Input: part model. Units: mm. Frame: model coordinates. Give positions to 0.01 mm unless a question says otherwise; leave off trailing zeros. Loops run counter-clockwise (first coordinate to the right, second up) from the corner with the lowest first, then second, coordinate; pieces in that order, holes last. Notation, with made-up numbers: (7, 4) -> (20, 4) arc R21 cw to (20, 33) -> close; hole circle Ø9 at (73.5, -12.75). An arc over 180 degrees is marked (long way). Use CSV: the item, a comma, the result in double quotes.
```python
from build123d import *

# Parameters (mm, degrees)
SKETCH1_R           = 4.5
BOSS_EXTRUDE1_DEPTH = 4.3
SKETCH2_R           = 3.9
CUT_EXTRUDE1_DEPTH  = 5.3
CHAMFER1_SIZE       = 0.2


with BuildPart() as part:
    # Sketch1 → Boss-Extrude1 (new body)
    with BuildSketch(Plane(origin=(0, 0, 0), x_dir=(1, 0, 0), z_dir=(0, 1, 0))):
        Circle(SKETCH1_R)
    extrude(amount=BOSS_EXTRUDE1_DEPTH)

    # Sketch2 → Cut-Extrude1 (cut, through all)
    with BuildSketch(Plane(origin=(0, 4.3, 0), x_dir=(1, 0, 0), z_dir=(0, 1, 0))):
        Circle(SKETCH2_R)
    extrude(amount=-CUT_EXTRUDE1_DEPTH, mode=Mode.SUBTRACT)

    # Chamfer1
    chamfer1_edges = [part.edges().sort_by_distance(p)[0] for p in [
        (-4.5, 0, 0),
    ]]
    chamfer(chamfer1_edges, length=CHAMFER1_SIZE)


solid = part.part
```
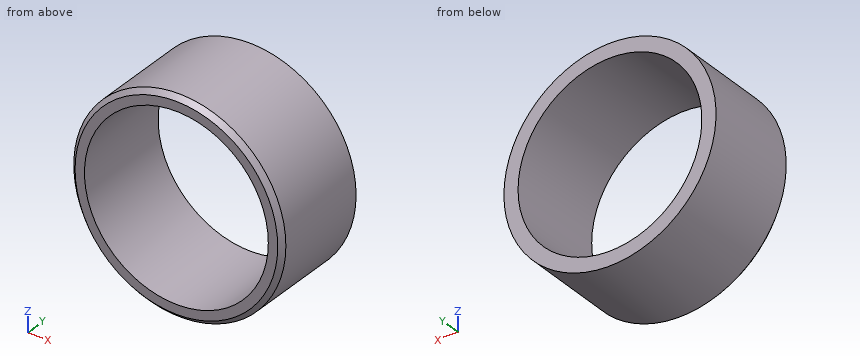
1) Section query B-B (x = 0). Return loops of the section in (y, z), then the cut area to 3 significant figures.
From the geometry:
outline,"(0, -4.3) -> (0.2, -4.5) -> (4.3, -4.5) -> (4.3, -3.9) -> (0, -3.9) -> close; (0, 3.9) -> (4.3, 3.9) -> (4.3, 4.5) -> (0.2, 4.5) -> (0, 4.3) -> close"
area,"5.12 mm^2"
2) Section query A-A (z = 0). Return loops of the section in (x, y).
From the geometry:
outline,"(-4.5, 0.2) -> (-4.3, 0) -> (-3.9, 0) -> (-3.9, 4.3) -> (-4.5, 4.3) -> close; (3.9, 0) -> (4.3, 0) -> (4.5, 0.2) -> (4.5, 4.3) -> (3.9, 4.3) -> close"
3) Section query C-C (y = 1.75). Return loops of the section in (x, z), then the cut area to 3 significant figures.
From the geometry:
outline,"circle Ø9 at (0, 0); hole circle Ø7.8 at (0, 0)"
area,"15.8 mm^2"
4) Ray query, line 1 (X direction, y = 3.4, z = 0); line 2 (X direction, y = 3.45, z = -1.5). Return the intervals inside material, ascending.
From the geometry:
line 1,"x = -4.5 to -3.9, 3.9 to 4.5"
line 2,"x = -4.24 to -3.6, 3.6 to 4.24"
5) Contact query for flat-ended pins moving along their axis: pin 1 (1 mm diameter, centred on x = -3.5, y = 2, fed in from +Z); pin 2 (5 mm diameter, centred on x = 0, z = 2.5, fed in from -Y); pin 3 (1.5 mm diameter, centred on y = 0.5, z = 2, fed in from -X). Output: stop coordinate, or through.
From the geometry:
pin 1,"stops at z = 3.35"
pin 2,"stops at y = 0"
pin 3,"stops at x = -4.32"
